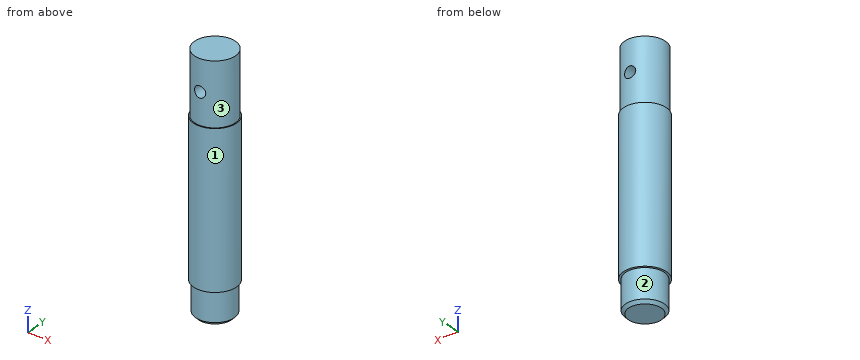
from build123d import *

# Parameters (mm, degrees)
SKETCH1_R           = 10
BOSS_EXTRUDE1_DEPTH = 57.5
SKETCH7_R           = 10
SKETCH7_R_2         = 9.5
CUT_EXTRUDE1_DEPTH  = 29
SKETCH10_W          = 2.65
SKETCH10_H          = 10


# Read off the part's stored shape, not the designer's step: M18x2.5 Machine Threads Stud1
with BuildPart() as part:
    # Sketch1 → Boss-Extrude1 (new, symmetric)
    with BuildSketch(Plane.XY):
        Circle(SKETCH1_R)
    extrude(amount=BOSS_EXTRUDE1_DEPTH, both=True)

    # M18x2.5 Machine Threads Stud1 outline → M18x2.5 Machine Threads Stud1 (revolve, cut)
    with BuildSketch(Plane.XZ):
        Polygon((7.626, -57.5), (10, -57.5), (10, -42.5), (9, -42.5), (9, -56.126), align=None)
    revolve(axis=Axis((0, 0, 0), (0, 0, 1)), mode=Mode.SUBTRACT)

    # Sketch7 → Cut-Extrude1 (cut)
    with BuildSketch(Plane.XY.offset(57.5)):
        Circle(SKETCH7_R)
        Circle(SKETCH7_R_2, mode=Mode.SUBTRACT)
    extrude(amount=-CUT_EXTRUDE1_DEPTH, mode=Mode.SUBTRACT)

    # Sketch10 → M5 Clearance Hole1 (revolve, cut)
    with BuildSketch(Plane(origin=(0, 0, 43), x_dir=(0, 0, -1), z_dir=(1, 0, 0))):
        with Locations((1.325, 5)):
            Rectangle(SKETCH10_W, SKETCH10_H)
    m5_clearance_hole1 = revolve(axis=Axis((0, -6.35, 43), (0, 1, 0)), mode=Mode.SUBTRACT)

    # Mirror2: M5 Clearance Hole1 across plane
    add(m5_clearance_hole1.mirror(Plane.ZX), mode=Mode.SUBTRACT)


solid = part.part
Here's how the part is built. I have some questions about the finished solid (model axes, mm). Face numbers are marked on the shaded views. A direction names the side the tool comes from. Round coordinates to 2 decimals unless told otherwise and drop trailing zeros. Loops run counter-clockwise (first coordinate to the right, second up) from the corner with the lowest first, then second, coordinate; pieces in that order, holes last. Notation, with made-up numbers: M 77,89 L 118,89 A28 ccw 118,110 Z; hole C -27,-8 d6. An arc over 180 degrees is marked long. Write each question's results on one line, items separated by ' | '. Start each with the question number.
(1) Will these pins go through, and if not, where does the flat tip stop? P1, Ø6, axis at x = 0, z = 43, coming from the -Y side; P2, Ø4, axis at y = 1, z = 42.5, coming from the +X side; P3, Ø8, axis at x = -5, z = 2.5, coming from the +Y side.
(2) I want a section at C-C (z = -2). Please give me the cut outline in (x, y), then the cut area to 3 significant figures.
(3) I want a section at A-A (x = 0). Please give me the cut outline in (y, z).
(4) On a 3-axis mill with a long thin cutter (end or side, diameter ignored), from which of +Z, -Z, +X, -X, +Y, -Y can I reach the whole of each face in a straight line? I mean the marked faces 1, 2 and 3. Say none if no direction works.
(5) If I drill on probe 1 along Z at (x, y) = (0, 4.5); probe 2 along X at (y, z) = (3, 43); probe 3 along Z at (x, y) = (-2, -7.5), over which ranges is the centre line in solid material (lowest first)? Write a range as from..to.
(6) I want a section at B-B (z = 43). Please give me the cut outline in (x, y).
Solved:
1) P1: stops at y = -9.5 | P2: stops at x = 9.5 | P3: stops at y = 9.95
2) outline: C 0,0 d20 | area: 314 mm²
3) outline: M -10,-42.5 L -9,-42.5 L -9,-56.13 L -7.63,-57.5 L 7.63,-57.5 L 9,-56.13 L 9,-42.5 L 10,-42.5 L 10,28.5 L 9.5,28.5 L 9.5,40.35 L -9.5,40.35 L -9.5,28.5 L -10,28.5 Z; M -9.5,45.65 L 9.5,45.65 L 9.5,57.5 L -9.5,57.5 Z
4) face 1: +Z, -Z | face 2: -Z | face 3: +Z
5) probe 1: z = -57.5..40.35, 45.65..57.5 | probe 2: x = -9.01..-2.65, 2.65..9.01 | probe 3: z = -57.36..41.26, 44.74..57.5
6) outline: M -2.65,-9.12 L -2.65,9.12 A9.5 ccw Z; M 2.65,-9.12 A9.5 ccw 2.65,9.12 Z
